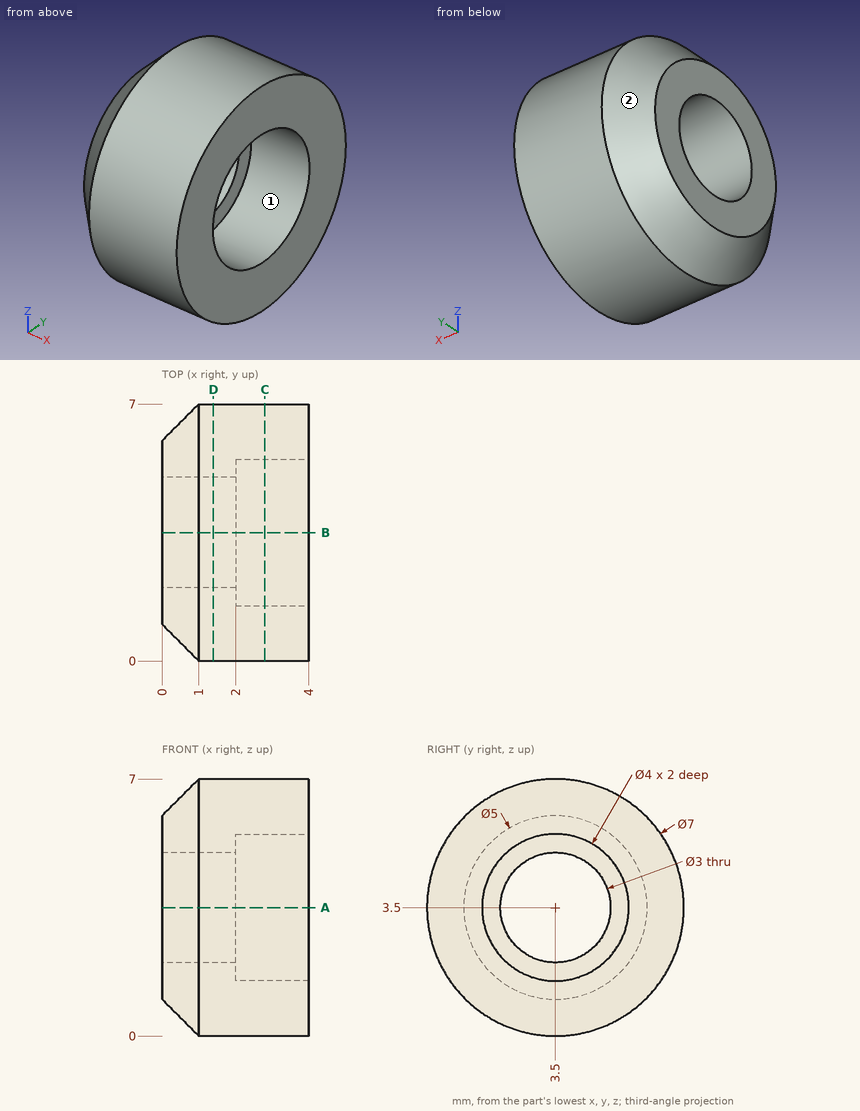
Design review of the part shown in the three views and the two pictorial views. Dimensions are in mm from the part's minimum x, y and z. A direction names the side the tool comes from. Coordinates: 2 decimals unless noted, no trailing zeros. Write each loop counter-clockwise with the first axis right and the second up, starting at its lowest first coordinate (ties: lowest second). Pieces come first, ordered by that corner, then holes. Notation, with made-up numbers: (66.25, 2) - (124.25, 2) arc R22 ccw to (124.25, 20) - close; hole circle Ø10 at (35, -23). An arc over 180 degrees is marked (long way). Write item = value, one per line.
(1) For P1, Ø1.2, axis at y = 3, z = 3, coming from the +X side, flat-tipped, find the tip position at first contact; note if it passes through.
Result sheet:
P1 = through
(2) Consider section D-D, the plane x = 1.4. Give the boundary of the cut face in (y, z).
Result sheet:
outline = circle Ø7 at (3.5, 3.5); hole circle Ø3 at (3.5, 3.5)
(3) Consider section A-A, the plane z = 3.5. Give the boundary of the cut face in (x, y).
Result sheet:
outline = (0, 1) - (1, 0) - (4, 0) - (4, 1.5) - (2, 1.5) - (2, 2) - (0, 2) - close; (0, 5) - (2, 5) - (2, 5.5) - (4, 5.5) - (4, 7) - (1, 7) - (0, 6) - close
(4) Machinability: for the marked faces 1 and 2, which of the approach directions +Z, -Z, +X, -X, +Y, -Y give a long, thin tool a straight path to every point of the face, cutting with its end or side? Answer none if there is none.
Result sheet:
face_1 = +X
face_2 = -X
(5) For line 1 (X direction, y = 4.5, z = 2); line 2 (Y direction, x = 1.25, z = 4.75), list the stretches that pass through material, from the lowest coordinate up. Write a range as [from, to].
Result sheet:
line_1 = [0, 2]
line_2 = [0.23, 2.67], [4.33, 6.77]
(6) Consider section C-C, the plane x = 2.8. Give the boundary of the cut face in (y, z), then the cut area to 3 significant figures.
Result sheet:
outline = circle Ø7 at (3.5, 3.5); hole circle Ø4 at (3.5, 3.5)
area = 25.9 mm^2
